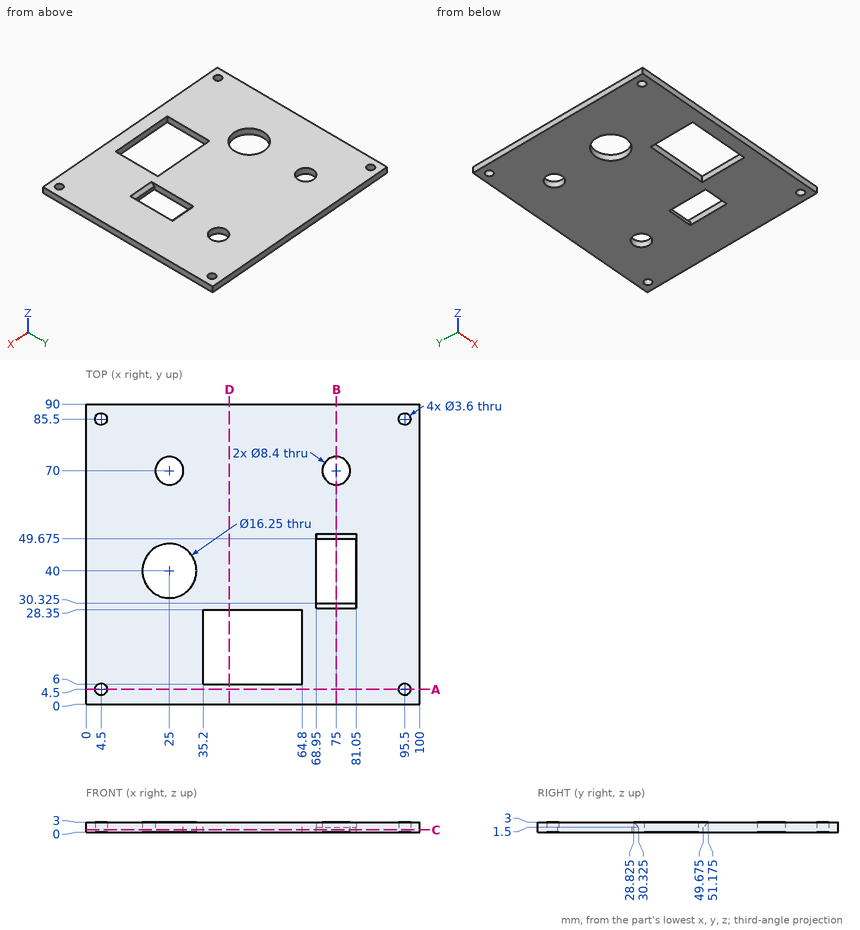
Answer from the drawing. Dimensions are ordinates in mm from the lowest x, y and z of the part. Give positions to 0.01 mm unless a question says otherwise; leave off trailing zeros. Order: outer loops, then holes, each group sorted by start corner. A loop starts at its lowest first (then second) coordinate and runs counter-clockwise, first axis right, second up. Notation, with made-up numbers: (3, 19.25) - (36, 19.25) arc R29 cw to (36, 57.25) - close; hole circle Ø8 at (77, -3.75). An arc over 180 degrees is marked (long way). One line per item, written item: value. Start each with the question number.
1. Section D-D, the plane x = 43 is taken. Write down the section's boundary in (y, z), then the cut area to 3 significant figures.
2. Section A-A, the plane y = 4.5 is taken. Write down the section's boundary in (x, z), then the cut area to 3 significant figures.
3. Section C-C, the plane z = 0.75 is taken. Count the separate pieces of the cut face and the enclosed holes in it, then the cut area to 3 significant figures.
4. This flat-tipped pin is pushed along its axis until it touches: pin 1 Ø3 at (x, y) = (4.5, 85.5) entering from -Z. Where does it stop, or does it pass through?
5. Consider line 1 (Y direction, x = 4.5, z = 1.1); line 2 (Y direction, x = 25, z = 0.8) (3 decimals); line 3 (Y direction, x = 50, z = 0.9). Determine where each line is inside the solid, lowest interval first.
6. Section B-B, the plane x = 75 is taken. Write down the section's boundary in (y, z) (3 decimals), then the cut area to 4 significant figures.
Filled sheet:
1. outline: (0, 0) - (6, 0) - (6, 3) - (0, 3) - close; (28.35, 0) - (90, 0) - (90, 3) - (28.35, 3) - close
1. area: 203 mm²
2. outline: (0, 0) - (2.7, 0) - (2.7, 3) - (0, 3) - close; (6.3, 0) - (93.7, 0) - (93.7, 3) - (6.3, 3) - close; (97.3, 0) - (100, 0) - (100, 3) - (97.3, 3) - close
2. area: 278 mm²
3. separate pieces: 1
3. enclosed holes: 9
3. area: 7,750 mm²
4. pin 1: through
5. line 1: 0 to 2.7, 6.3 to 83.7, 87.3 to 90
5. line 2: 0 to 31.875, 48.125 to 65.8, 74.2 to 90
5. line 3: 0 to 6, 28.35 to 90
6. outline: (0, 0) - (30.325, 0) - (30.325, 1.5) - (28.825, 3) - (0, 3) - close; (49.675, 0) - (65.8, 0) - (65.8, 3) - (51.175, 3) - (49.675, 1.5) - close; (74.2, 0) - (90, 0) - (90, 3) - (74.2, 3) - close
6. area: 184.5 mm²
